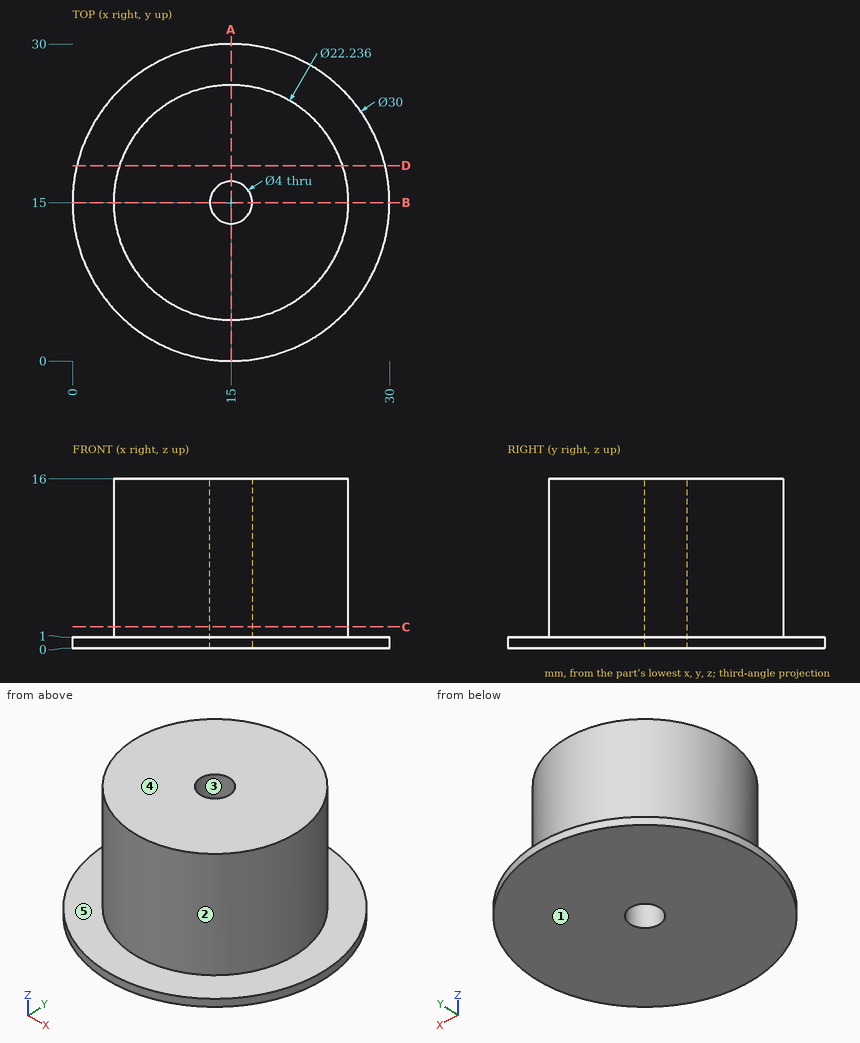
Geometry: see drawing. Coordinates: mm, zero at the bounding-box minimum. A direction names the side the tool comes from. Round coordinates to 2 decimals unless told otherwise and drop trailing zeros. Order: outer loops, then holes, each group sorted by start corner. A loop starts at its lowest first (then second) coordinate and runs counter-clockwise, first axis right, second up. Notation, with made-up numbers: (65, 44) - (87, 44) arc R21 ccw to (87, 63) - close; hole circle Ø10 at (0.5, 32). An arc over 180 degrees is marked (long way). Use a Markdown table: item, result. Add a question column.
1. Mould query, pull axis Y, two halves, no side actions, for the marked faces 1, 2 and 3. Classes: +Y half, -Y half, draft (parallel to the pull), parting line (faces both ways), or undercut.
2. First-contact query: pin 1 (1 mm diameter, centred on x = 23.5, y = 15, fed in from -Z); pin 2 (2 mm diameter, centred on x = 16.5, z = 10, fed in from +Y); pin 3 (6 mm diameter, centred on y = 3, z = 7.5, fed in from -X). Flat tips, straight axial feed; report the tip coordinate or a pass-through.
3. Section query A-A (x = 15). Return the cut outline in (y, z), then the cut area to 3 significant figures.
4. Line query: probe 1 along Y at (x, z) = (15, 9.75); probe 2 along Z at (x, y) = (3.5, 7.5); probe 3 along X at (y, z) = (16.5, 8.5). Output: solid intervals per line, ascending.
5. Section query C-C (z = 2). Return the cut outline in (x, y), then the cut area to 3 significant figures.
6. Set-up query: the marked faces 4 and 5. Return all of +Z, -Z, +X, -X, +Y, -Y with unobstructed straight access to the full face (end or side cutting, diameter ignored); none if empty.
7. Section query D-D (y = 18.5). Return the cut outline in (x, z), then the cut area to 3 significant figures.
Derived:
| question | item | result |
|---|---|---|
| 1 | face 1 | draft |
| 1 | face 2 | parting line |
| 1 | face 3 | undercut |
| 2 | pin 1 | z = 0 |
| 2 | pin 2 | y = 26.11 |
| 2 | pin 3 | x = 8.47 |
| 3 | outline | (0, 0) - (13, 0) - (13, 16) - (3.88, 16) - (3.88, 1) - (0, 1) - close; (17, 0) - (30, 0) - (30, 1) - (26.12, 1) - (26.12, 16) - (17, 16) - close |
| 3 | area | 300 mm2 |
| 4 | probe 1 | 3.88 to 13, 17 to 26.12 |
| 4 | probe 2 | 0 to 1 |
| 4 | probe 3 | 3.98 to 13.68, 16.32 to 26.02 |
| 5 | outline | circle Ø22.24 at (15, 15); hole circle Ø4 at (15, 15) |
| 5 | area | 376 mm2 |
| 6 | face 4 | +Z, +X, -X, +Y, -Y |
| 6 | face 5 | +Z |
| 7 | outline | (0.41, 0) - (29.59, 0) - (29.59, 1) - (25.55, 1) - (25.55, 16) - (4.45, 16) - (4.45, 1) - (0.41, 1) - close |
| 7 | area | 346 mm2 |
